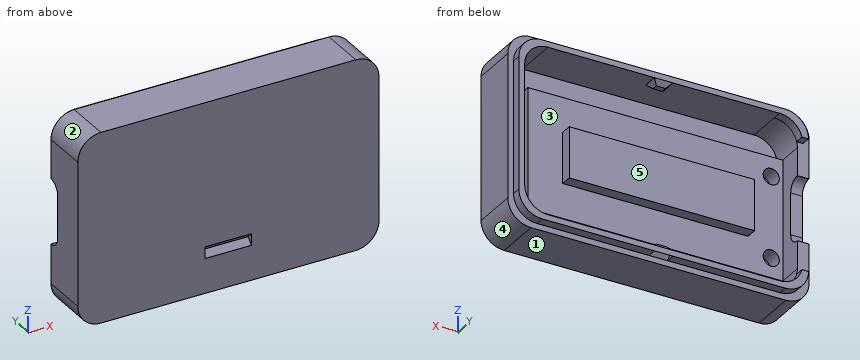
from build123d import *

# Parameters (mm, degrees)
SKETCH2_W                 = 55
SKETCH2_H                 = 26
BOSS_EXTRUDE3_DEPTH       = 4.55
SKETCH4_W                 = 40
SKETCH4_H                 = 11
BOSS_EXTRUDE5_DEPTH       = 7
BOSS_EXTRUDE6_DEPTH       = 2.5
BOSS_EXTRUDE7_DEPTH       = 10
BOSS_EXTRUDE9_DEPTH       = 2
BOSS_EXTRUDE10_DEPTH      = 2
BOSS_EXTRUDE10_DEPTH_BACK = 2
CUT_EXTRUDE2_DEPTH        = 2
CUT_EXTRUDE2_DEPTH_BACK   = 2
CUT_EXTRUDE3_DEPTH        = 4
CUT_EXTRUDE4_DEPTH        = 5
CUT_EXTRUDE4_DEPTH_BACK   = 5
CUT_EXTRUDE6_DEPTH        = 10
SKETCH14_R                = 1.75
CUT_EXTRUDE7_DEPTH        = 4


with BuildPart() as part:
    # Sketch2 → Boss-Extrude3 (new body)
    with BuildSketch(Plane(origin=(0, 0, 0), x_dir=(1, 0, 0), z_dir=(0, 1, 0))):
        with Locations((27.5, 13)):
            Rectangle(SKETCH2_W, SKETCH2_H)
    extrude(amount=BOSS_EXTRUDE3_DEPTH)

    # Sketch4 → Boss-Extrude5 (add)
    with BuildSketch(Plane(origin=(0, 0, 0), x_dir=(1, 0, 0), z_dir=(0, 1, 0))):
        with Locations((27.5, 13)):
            Rectangle(SKETCH4_W, SKETCH4_H)
    extrude(amount=BOSS_EXTRUDE5_DEPTH)

    # Sketch5 → Boss-Extrude6 (add)
    with BuildSketch(Plane(origin=(0, 0, 0), x_dir=(1, 0, 0), z_dir=(0, 1, 0))):
        with BuildLine():
            Line((5, 31), (55, 31))
            ThreePointArc((55, 31), (58.535533906, 29.535533906), (60, 26))
            Line((60, 26), (60, 0))
            ThreePointArc((60, 0), (58.535533906, -3.535533906), (55, -5))
            Line((55, -5), (5, -5))
            ThreePointArc((5, -5), (1.464466094, -3.535533906), (0, 0))
            Line((0, 0), (0, 26))
            ThreePointArc((0, 26), (1.464466094, 29.535533906), (5, 31))
        make_face()
    extrude(amount=BOSS_EXTRUDE6_DEPTH)

    # Sketch6 → Boss-Extrude7 (add)
    with BuildSketch(Plane(origin=(0, 0, 0), x_dir=(1, 0, 0), z_dir=(0, 1, 0))):
        with BuildLine():
            Line((2.5, 33.5), (57.5, 33.5))
            ThreePointArc((57.5, 33.5), (61.035533906, 32.035533906), (62.5, 28.5))
            Line((62.5, 28.5), (62.5, -2.5))
            ThreePointArc((62.5, -2.5), (61.035533906, -6.035533906), (57.5, -7.5))
            Line((57.5, -7.5), (2.5, -7.5))
            ThreePointArc((2.5, -7.5), (-1.035533906, -6.035533906), (-2.5, -2.5))
            Line((-2.5, -2.5), (-2.5, 28.5))
            ThreePointArc((-2.5, 28.5), (-1.035533906, 32.035533906), (2.5, 33.5))
        make_face()
        with BuildLine():
            Line((5, 31), (55, 31))
            ThreePointArc((55, 31), (58.535533906, 29.535533906), (60, 26))
            Line((60, 26), (60, 0))
            ThreePointArc((60, 0), (58.535533906, -3.535533906), (55, -5))
            Line((55, -5), (5, -5))
            ThreePointArc((5, -5), (1.464466094, -3.535533906), (0, 0))
            Line((0, 0), (0, 26))
            ThreePointArc((0, 26), (1.464466094, 29.535533906), (5, 31))
        make_face(mode=Mode.SUBTRACT)
    extrude(amount=BOSS_EXTRUDE7_DEPTH)

    # Sketch8 → Boss-Extrude9 (add)
    with BuildSketch(Plane(origin=(0, 10, 0), x_dir=(1, 0, 0), z_dir=(0, 1, 0))):
        with BuildLine():
            Line((56.25, 32.25), (3.75, 32.25))
            ThreePointArc((3.75, 32.25), (0.214466094, 30.785533906), (-1.25, 27.25))
            Line((-1.25, 27.25), (0.158770817, 27.25))
            ThreePointArc((0.158770817, 27.25), (1.938137822, 29.952847075), (5, 31))
            Line((5, 31), (55, 31))
            ThreePointArc((55, 31), (58.535533906, 29.535533906), (60, 26))
            Line((60, 26), (60, 0))
            ThreePointArc((60, 0), (58.535533906, -3.535533906), (55, -5))
            Line((55, -5), (5, -5))
            ThreePointArc((5, -5), (1.938137822, -3.952847075), (0.158770817, -1.25))
            Line((0.158770817, -1.25), (-1.25, -1.25))
            ThreePointArc((-1.25, -1.25), (0.214466094, -4.785533906), (3.75, -6.25))
            Line((3.75, -6.25), (56.25, -6.25))
            ThreePointArc((56.25, -6.25), (59.785533906, -4.785533906), (61.25, -1.25))
            Line((61.25, -1.25), (61.25, 27.25))
            ThreePointArc((61.25, 27.25), (59.785533906, 30.785533906), (56.25, 32.25))
        make_face()
    extrude(amount=BOSS_EXTRUDE9_DEPTH)

    # Sketch9 → Boss-Extrude10 (add, two sides: drawn at the far end of the back side and taken through both)
    with BuildSketch(Plane(origin=(30, 0, 0), x_dir=(0, 0, -1), z_dir=(1, 0, 0)).offset(-BOSS_EXTRUDE10_DEPTH_BACK)):
        Polygon((-5, 12), (-4, 11), (-4, 9.75), (-5, 8.75), align=None)
        Polygon((31, 12), (30, 11), (30, 9.75), (31, 8.75), align=None)
    extrude(amount=BOSS_EXTRUDE10_DEPTH + BOSS_EXTRUDE10_DEPTH_BACK)

    # Sketch10 → Cut-Extrude2 (cut, two sides: drawn at the far end of the back side and taken through both)
    with BuildSketch(Plane(origin=(30, 0, 0), x_dir=(0, 0, -1), z_dir=(1, 0, 0)).offset(-CUT_EXTRUDE2_DEPTH_BACK)):
        Polygon((-6.25, 12), (-5.249964226, 10.999964226), (-6.25, 10), align=None)
        Polygon((32.25, 12), (31.25, 11), (32.25, 10), align=None)
    extrude(amount=CUT_EXTRUDE2_DEPTH + CUT_EXTRUDE2_DEPTH_BACK, mode=Mode.SUBTRACT)

    # Sketch11 → Cut-Extrude3 (cut)
    with BuildSketch(Plane(origin=(0, 12, 0), x_dir=(1, 0, 0), z_dir=(0, 1, 0))):
        Polygon((32, 31), (32, 30), (31, 30), align=None)
        Polygon((28, 31), (28, 30), (29, 30), align=None)
        Polygon((28, -5), (28, -4), (29, -4), align=None)
        Polygon((32, -5), (32, -4), (31, -4), align=None)
    extrude(amount=-CUT_EXTRUDE3_DEPTH, mode=Mode.SUBTRACT)

    # Sketch12 → Cut-Extrude4 (cut, two sides: drawn at the far end of the back side and taken through both)
    with BuildSketch(Plane(origin=(30, 0, 0), x_dir=(0, 0, -1), z_dir=(1, 0, 0)).offset(-CUT_EXTRUDE4_DEPTH_BACK)):
        Polygon((23.5, 0), (26, 0), (24.75, 1.25), align=None)
    extrude(amount=CUT_EXTRUDE4_DEPTH + CUT_EXTRUDE4_DEPTH_BACK, mode=Mode.SUBTRACT)

    # Sketch7 → Cut-Extrude6 (cut)
    with BuildSketch(Plane(origin=(0, 0, 0), x_dir=(0, 0, -1), z_dir=(1, 0, 0))):
        with BuildLine():
            Line((13, 10), (19.990431296, 10))
            ThreePointArc((19.990431296, 10), (19.261010337, 11.760977972), (17.500032365, 12.490398932))
            Line((17.500032365, 12.490398932), (8.499967635, 12.490398932))
            ThreePointArc((8.499967635, 12.490398932), (6.738989663, 11.760977972), (6.009568704, 10))
            Line((6.009568704, 10), (13, 10))
        make_face()
        with BuildLine():
            ThreePointArc((17.500032365, 7.509601068), (19.261010337, 8.239022028), (19.990431296, 10))
            Line((19.990431296, 10), (13, 10))
            Line((13, 10), (6.009568704, 10))
            ThreePointArc((6.009568704, 10), (6.738989663, 8.239022028), (8.499967635, 7.509601068))
            Line((8.499967635, 7.509601068), (17.500032365, 7.509601068))
        make_face()
    extrude(amount=-CUT_EXTRUDE6_DEPTH, mode=Mode.SUBTRACT)

    # Sketch14 → Cut-Extrude7 (cut)
    with BuildSketch(Plane(origin=(0, 5, 0), x_dir=(1, 0, 0), z_dir=(0, 1, 0))):
        with Locations(Location((2.5, 21.75, 0), (0, 0, 270))):
            Circle(SKETCH14_R)
        with Locations(Location((2.5, 4.25, 0), (0, 0, 270))):
            Circle(SKETCH14_R)
    extrude(amount=-CUT_EXTRUDE7_DEPTH, mode=Mode.SUBTRACT)


solid = part.part
Check sheet for the modelled part. Datum: model origin and axes. Units: mm. Face numbers are marked on the shaded views. A direction names the side the tool comes from. Round coordinates to 2 decimals unless told otherwise and drop trailing zeros. Loops run counter-clockwise (first coordinate to the right, second up) from the corner with the lowest first, then second, coordinate; pieces in that order, holes last. Notation, with made-up numbers: (39, -38) - (54, -38) arc R37 cw to (54, 1) - close; hole circle Ø5 at (16, 76.25). An arc over 180 degrees is marked (long way). Answer as CSV lines item,"result". Start each with the question number.
Item 1: Section check B-B (x = 20). Record the boundary of the cut face in (y, z).
Item 2: Depth check by flat-ended pin: P1, Ø9, axis at x = 34.5, z = -12, coming from the +Y side; P2, Ø5.5, axis at x = 2.5, z = -21.75, coming from the +Y side; P3, Ø0.7, axis at x = -0.5, y = 11.5, coming from the -Z side; P4, Ø10, axis at x = 32.5, z = -7.5, coming from the -Y side. Enter the tip coordinate at first touch or a pass-through.
Item 3: Section check C-C (z = -10.5). Record the boundary of the cut face in (x, y).
Item 4: Section check A-A (z = -4.25). Record the boundary of the cut face in (x, y), and give its area (3 significant figures).
Item 5: Release check for a two-part mould opening along Z. For the marked faces 1, 2 and 3 record: +Z half, -Z half, draft (parallel to the pull), parting line (faces both ways), or undercut.
Item 6: Scan lines: line 1 (Z direction, x = 7, y = 4); line 2 (X direction, y = 3.55, z = -21.75); line 3 (Z direction, x = 8, y = 5.5). Record each from-to range of solid material in increasing order. Write a range as [from, to].
Item 7: Set-up check for the marked faces 4 and 5: record each of +Z, -Z, +X, -X, +Y, -Y from which the full face is reachable in a straight line by a thin tool's end or side.
Report:
1,outline,"(0, -33.5) - (10, -33.5) - (10, -32.25) - (12, -32.25) - (12, -31) - (2.5, -31) - (2.5, -26) - (4.55, -26) - (4.55, -18.5) - (7, -18.5) - (7, -7.5) - (4.55, -7.5) - (4.55, 0) - (2.5, 0) - (2.5, 5) - (12, 5) - (12, 6.25) - (10, 6.25) - (10, 7.5) - (0, 7.5) - close"
2,P1,"stops at y = 7"
2,P2,"stops at y = 10"
2,P3,"stops at z = -30.38"
2,P4,"stops at y = 0"
3,outline,"(-2.5, 0) - (62.5, 0) - (62.5, 10) - (61.25, 10) - (61.25, 12) - (60, 12) - (60, 2.5) - (55, 2.5) - (55, 4.55) - (47.5, 4.55) - (47.5, 7) - (7.5, 7) - (7.5, 4.55) - (0, 4.55) - (0, 7.51) - (-2.5, 7.51) - close"
4,outline,"(-2.5, 0) - (62.5, 0) - (62.5, 10) - (61.25, 10) - (61.25, 12) - (60, 12) - (60, 2.5) - (55, 2.5) - (55, 4.55) - (4.25, 4.55) - (4.25, 1) - (0.75, 1) - (0.75, 4.55) - (0, 4.55) - (0, 10) - (-2.5, 10) - close"
4,area,"303 mm2"
5,face 1,"-Z half"
5,face 2,"+Z half"
5,face 3,"undercut"
6,line 1,"z = [-33.5, -31], [-26, 0], [5, 7.5]"
6,line 2,"x = [-2.5, 0.75], [4.25, 55], [60, 62.5]"
6,line 3,"z = [-33.5, -31], [-18.5, -7.5], [5, 7.5]"
7,face 4,"-Z, +X, +Y, -Y"
7,face 5,"+Y"
